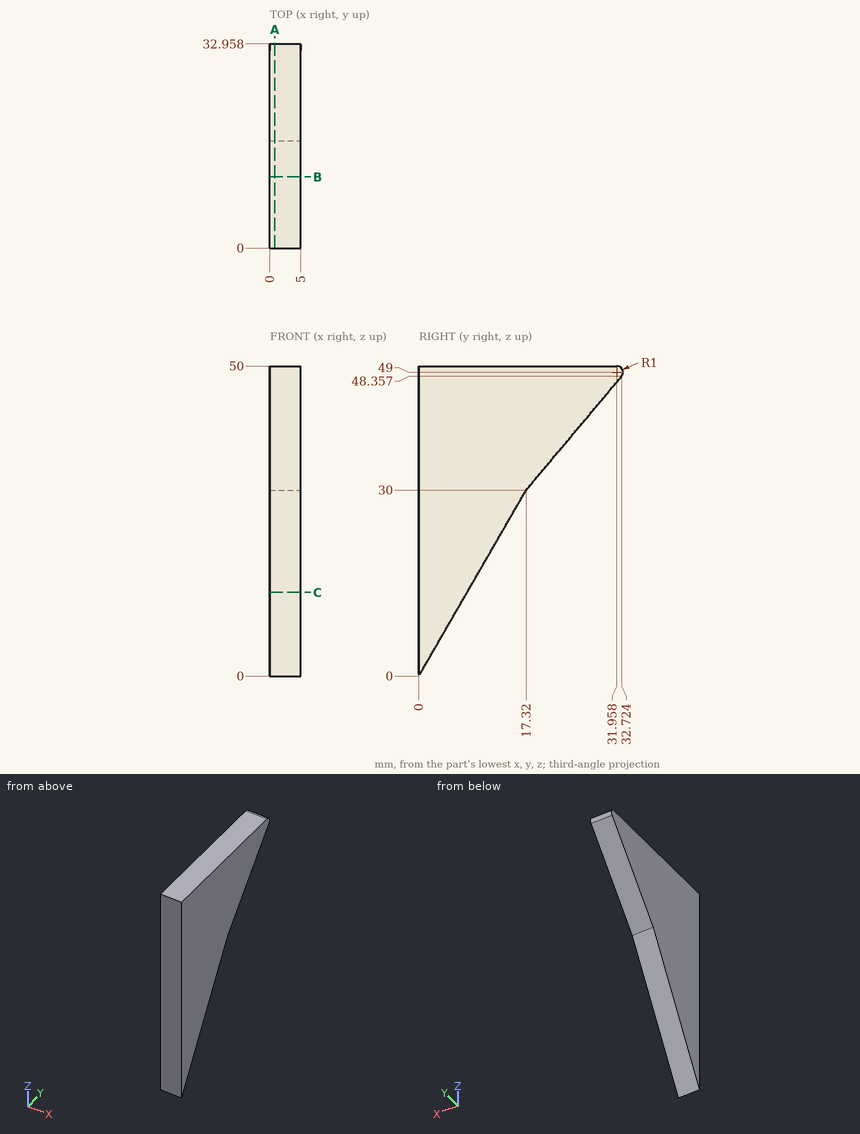
Part print with two shaded views. Sizes in mm from the minimum x, y, z corner. Coordinates: 2 decimals unless noted, no trailing zeros. Write each loop counter-clockwise with the first axis right and the second up, starting at its lowest first coordinate (ties: lowest second). Pieces come first, ordered by that corner, then holes.
1. Band-saw the part on A-A, the plane x = 0.8. Give the cut face in (y, z) (1 decimal), and give its area (3 significant figures).
Answer block:
outline: (0, 0) - (17.3, 30) - (32.7, 48.4) arc R1 ccw to (32, 50) - (0, 50) - close
area: 773 mm2
2. Drill centre lines: probe 1 along Y at (x, z) = (2.95, 18.5); probe 2 along Z at (x, y) = (4.6, 28) (1 decimal); probe 3 along Z at (x, y) = (0.9, 11.5) (1 decimal). Where is each one in solid material? Low to high.
Answer block:
probe 1: y = 0 to 10.68
probe 2: z = 42.7 to 50
probe 3: z = 19.9 to 50
3. Band-saw the part on B-B, the plane y = 11.5. Give the cut face in (x, z).
Answer block:
outline: (0, 19.92) - (5, 19.92) - (5, 50) - (0, 50) - close
4. Band-saw the part on C-C, the plane z = 13.5. Give the cut face in (x, y) (1 decimal).
Answer block:
outline: (0, 0) - (5, 0) - (5, 7.8) - (0, 7.8) - close
5. Drop flat-ended pins along their axis: pin 1 (2 mm diameter, centred on x = 2, z = 38, fed in from +Y); pin 2 (6 mm diameter, centred on y = 24.5, z = 32, fed in from +X). Give the stop position or say it passes through.
Answer block:
pin 1: stops at y = 24.87
pin 2: passes through
